from build123d import *

# Parameters (mm, degrees)
PAD_DEPTH = 5


with BuildPart() as part:
    # Sketch → Pad (new body)
    with BuildSketch(Plane.XY):
        Polygon((60.621778, 35), (0, 70), (-60.621778, 35), (-60.621778, -35), (0, -70), (60.621778, -35), align=None)
        Polygon((-17.320508, 50), (34.641016, 20), (17.320508, 10), (-34.641016, 40), (-51.961524, 30), (-51.961524, -30), (-34.641016, -40), (-34.641016, 20), (-17.320508, 10), (-17.320508, -50), (0, -60), (17.320508, -50), (0, -42.427157), (0, -15), (51.961524, 15), (51.961524, 30), (0, 60), align=None, mode=Mode.SUBTRACT)
        Polygon((51.961524, -5), (10, -29.226497), (34.641016, -40), (51.961524, -30), align=None, mode=Mode.SUBTRACT)
    extrude(amount=PAD_DEPTH)


solid = part.part
Can you work these out from the model? Positions are in its coordinate system, mm. A direction names the side the tool comes from. Coordinates: 2 decimals unless noted, no trailing zeros. Write each loop counter-clockwise with the first axis right and the second up, starting at its lowest first coordinate (ties: lowest second). Pieces come first, ordered by that corner, then holes. Notation, with made-up numbers: (10, -25) - (29, -25) arc R33 ccw to (29, 7) - close; hole circle Ø2 at (23, -30). An arc over 180 degrees is marked (long way). Return JSON: item names as keys, results as strings. Group by question number.
Item 1: If we section it at D-D (x = -9): Write out the boundary of the cut face in (y, z).
Item 2: Please list where these lines run through material, in increasing order: probe 1 along X at (y, z) = (-12.5, 0.4); probe 2 along Y at (x, z) = (28.5, 3.25); probe 3 along X at (y, z) = (-9.5, 4.3).
Item 3: Which directions (+Z, -Z, +X, -X, +Y, -Y) give clear straight access to the entire face, cutting with the end or side of a thin tool? Please do faces 1 (the face through (-43.42, -34.93, 2.46)), 2 (the face through (30.735, 52.255, 2.465)).
Item 4: If we section it at B-B (x = 22.5): Write out the boundary of the cut face in (y, z).
Item 5: If we section it at A-A (z = 2.8): Write out the boundary of the cut face in (x, y), then the cut area to 3 significant figures.
Item 6: If we section it at C-C (y = -31.5): Write out the boundary of the cut face in (x, z), then the cut area to 3 significant figures.
Item 7: We'd pull the mould along X, two halves only. Please class faces 3 (the face through (13, -15, 0)), 4 (the face through (29.887, -52.745, 2.465)), 5 (the face through (-8.54, 55.07, 2.46)), 6 (the face through (43.18, -35.07, 2.46)): pulls with the +X half, pulls with the -X half, needs draft (parallel to the pull), parting line crosses it, or undercut.
Return value:
{
 "1": {"outline": "(-64.8, 0) - (-54.8, 0) - (-54.8, 5) - (-64.8, 5) - close; (25.2, 0) - (45.2, 0) - (45.2, 5) - (25.2, 5) - close; (54.8, 0) - (64.8, 0) - (64.8, 5) - (54.8, 5) - close"},
 "2": {"probe 1": "x = -60.62 to -51.96, -34.64 to -17.32, 4.33 to 38.97, 51.96 to 60.62", "probe 2": "y = -53.55 to -37.32, -18.55 to 1.45, 16.45 to 23.55, 43.55 to 53.55", "probe 3": "x = -60.62 to -51.96, -34.64 to -17.32, 9.53 to 44.17, 51.96 to 60.62"},
 "3": {"face 1": "+Z, -Z", "face 2": "+Z, -Z, +X, +Y"},
 "4": {"outline": "(-57.01, 0) - (-34.69, 0) - (-34.69, 5) - (-57.01, 5) - close; (-22.01, 0) - (-2.01, 0) - (-2.01, 5) - (-22.01, 5) - close; (12.99, 0) - (27.01, 0) - (27.01, 5) - (12.99, 5) - close; (47.01, 0) - (57.01, 0) - (57.01, 5) - (47.01, 5) - close"},
 "5": {"outline": "(-60.62, -35) - (0, -70) - (60.62, -35) - (60.62, 35) - (0, 70) - (-60.62, 35) - close; hole (-51.96, -30) - (-34.64, -40) - (-34.64, 20) - (-17.32, 10) - (-17.32, -50) - (0, -60) - (17.32, -50) - (0, -42.43) - (0, -15) - (51.96, 15) - (51.96, 30) - (0, 60) - (-17.32, 50) - (34.64, 20) - (17.32, 10) - (-34.64, 40) - (-51.96, 30) - close; hole (10, -29.23) - (34.64, -40) - (51.96, -30) - (51.96, -5) - close", "area": "6,900 mm^2"},
 "6": {"outline": "(-60.62, 0) - (-49.36, 0) - (-49.36, 5) - (-60.62, 5) - close; (-34.64, 0) - (-17.32, 0) - (-17.32, 5) - (-34.64, 5) - close; (0, 0) - (15.2, 0) - (15.2, 5) - (0, 5) - close; (49.36, 0) - (60.62, 0) - (60.62, 5) - (49.36, 5) - close", "area": "275 mm^2"},
 "7": {"face 3": "needs draft", "face 4": "pulls with the +X half", "face 5": "undercut", "face 6": "undercut"}
}
